Verification items for this drawing (mm, ordinates from the low corner). Round coordinates to 2 decimals unless told otherwise and drop trailing zeros. Order: outer loops, then holes, each group sorted by start corner. A loop starts at its lowest first (then second) coordinate and runs counter-clockwise, first axis right, second up. Notation, with made-up numbers: (51, -34) -> (84, -34) arc R17 cw to (84, -10) -> close; hole circle Ø3 at (54, -31.5). An arc over 180 degrees is marked (long way). Answer in a Markdown table with one row per item. Add a question column.
1. Sectioned sample at C-C, the plane x = 28. Record the boundary of the cut face in (y, z).
2. Depth check by flat-ended pin: P1, Ø15, axis at x = 21.5, z = 49.5, coming from the +Y side; P2, Ø8, axis at x = 28.5, y = 11, coming from the -Z side; P3, Ø8, axis at y = 8, z = 137, coming from the -X side; P4, Ø7, axis at x = 17.5, y = 8, coming from the +Z side. Enter the tip coordinate at first touch or a pass-through.
3. Draft check along Z on the marked faces 1, 2 and 3. Enter one of: +Z half, -Z half, draft (parallel to the pull), parting line (faces both ways), or undercut.
4. Material ranges on L1, parallel to X at y = 10, z = 29; L2, parallel to Z at x = 32.5, y = 8.75; L3, parallel to Z at x = 3, y = 3.25, recorded low to high. Write a range as from..to.
5. Sectioned sample at A-A, the plane y = 13. Record the boundary of the cut face in (x, z).
6. Sectioned sample at B-B, the plane z = 82.5. Record the boundary of the cut face in (x, y).
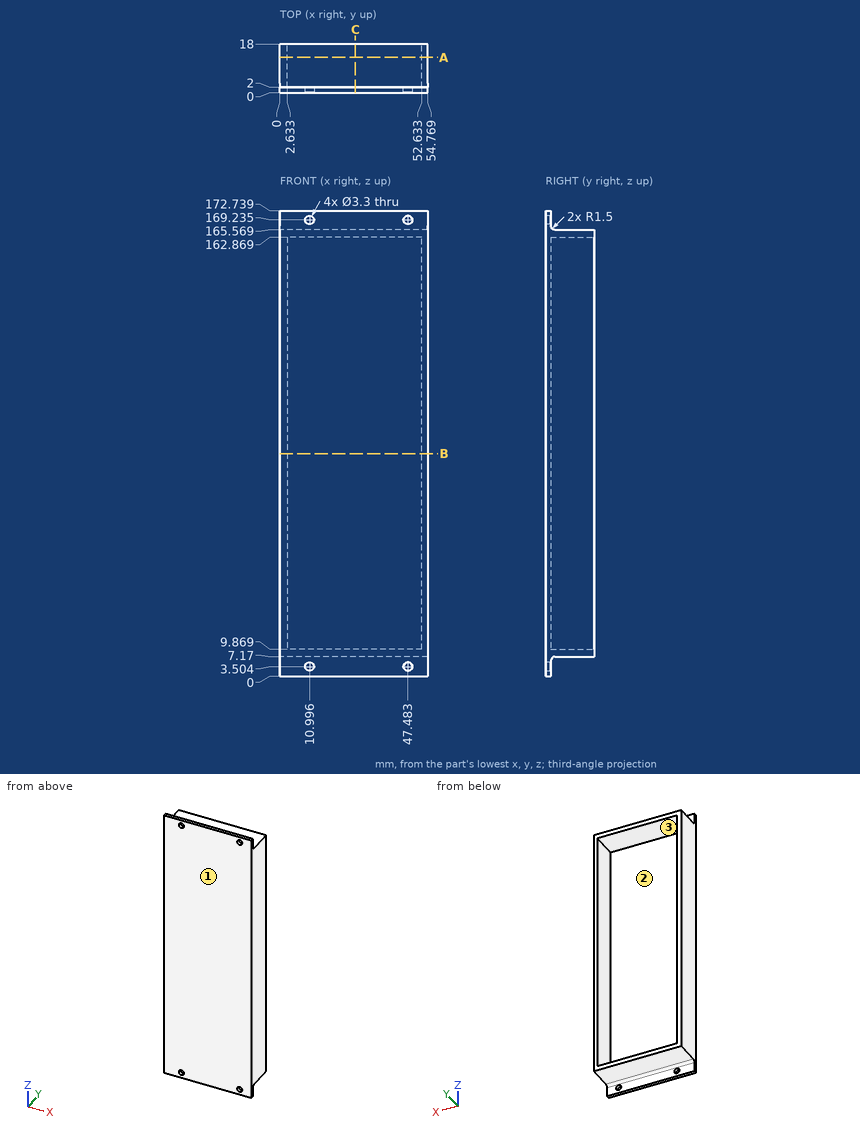
Answer key:
| question | item | result |
|---|---|---|
| 1 | outline | (0, 0) -> (2, 0) -> (2, 5.67) arc R1.5 cw to (3.5, 7.17) -> (18, 7.17) -> (18, 9.87) -> (2, 9.87) -> (2, 162.87) -> (18, 162.87) -> (18, 165.57) -> (3.5, 165.57) arc R1.5 cw to (2, 167.07) -> (2, 172.74) -> (0, 172.74) -> close |
| 2 | P1 | stops at y = 2 |
| 2 | P2 | stops at z = 7.17 |
| 2 | P3 | stops at x = 0 |
| 2 | P4 | stops at z = 165.57 |
| 3 | face 1 | draft |
| 3 | face 2 | undercut |
| 3 | face 3 | undercut |
| 4 | L1 | x = 0..2.63, 52.63..54.77 |
| 4 | L2 | z = 7.17..9.87, 162.87..165.57 |
| 4 | L3 | z = 7.15..9.87, 162.87..165.59 |
| 5 | outline | (0, 7.17) -> (54.77, 7.17) -> (54.77, 165.57) -> (0, 165.57) -> close; hole (2.63, 9.87) -> (52.63, 9.87) -> (52.63, 162.87) -> (2.63, 162.87) -> close |
| 6 | outline | (0, 0) -> (54.77, 0) -> (54.77, 18) -> (52.63, 18) -> (52.63, 2) -> (2.63, 2) -> (2.63, 18) -> (0, 18) -> close |
